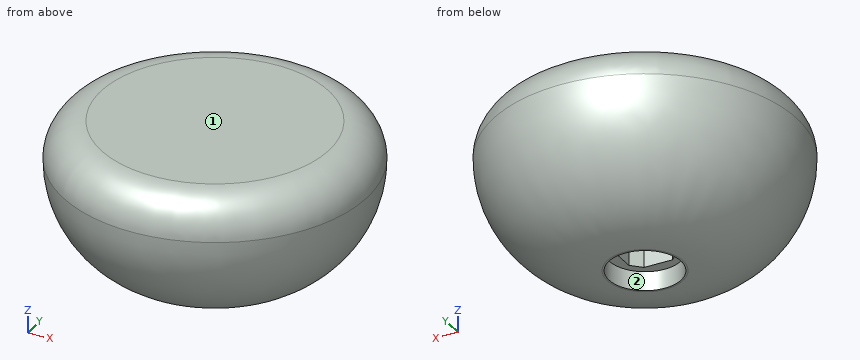
from build123d import *

# Parameters (mm, degrees)
EXTRUDE_3_OUTLINE_R   = 8
EXTRUDE_3_OUTLINE_R_2 = 1.904306864
EXTRUDE_3_OUTLINE_R_3 = 1.884306864
EXTRUDE_3_DEPTH       = 4
EXTRUDE_START         = -1
SKETCH_4_3_R          = 8
SKETCH_4_3_R_2        = 1.904306864
EXTRUDE_4_DEPTH       = 1
SKETCH_5_R            = 8
EXTRUDE_5_DEPTH       = 3
FILLET_3_R            = 2
FILLET_4_R            = 6


# Read off the part's stored shape, not the designer's step: 凸台-拉伸3
with BuildPart() as part:
    # 凸台-拉伸3 outline → 凸台-拉伸3 (new body)
    # profile 1 of 2: a face of its own
    with BuildSketch(Plane.XY.offset(15.156605354)):
        with Locations((62.088098202, 10.274465036)):
            Circle(EXTRUDE_3_OUTLINE_R)
        with Locations((62.088098202, 10.274465036)):
            Circle(EXTRUDE_3_OUTLINE_R_2, mode=Mode.SUBTRACT)
    # profile 2 of 2: a face of its own
    with BuildSketch(Plane.XY.offset(15.156605354)):
        with Locations((62.088098202, 10.274465036)):
            Circle(EXTRUDE_3_OUTLINE_R_3)
        Polygon((62.846382474, 11.544465036), (63.358098202, 11.032749307), (63.358098202, 9.516180765), (62.846382474, 9.004465036), (61.329813931, 9.004465036), (60.818098202, 9.516180765), (60.818098202, 11.032749307), (61.329813931, 11.544465036), align=None, mode=Mode.SUBTRACT)
    extrude(amount=EXTRUDE_3_DEPTH)

    # 草图4<3> → 凸台-拉伸4 (add)
    with BuildSketch(Plane.XY.offset(15.156605354).offset(EXTRUDE_START)):
        with Locations((62.088098202, 10.274465036)):
            Circle(SKETCH_4_3_R)
        with Locations((62.088098202, 10.274465036)):
            Circle(SKETCH_4_3_R_2, mode=Mode.SUBTRACT)
    extrude(amount=EXTRUDE_4_DEPTH)

    # 草图5 → 凸台-拉伸5 (add)
    with BuildSketch(Plane.XY.offset(19.156605354)):
        with Locations((62.088098202, 10.274465036)):
            Circle(SKETCH_5_R)
    extrude(amount=EXTRUDE_5_DEPTH)

    # 圆角3
    fillet_3_edges = [part.edges().sort_by_distance(p)[0] for p in [
        (54.088098202, 10.274465036, 22.156605354),
    ]]
    fillet(fillet_3_edges, radius=FILLET_3_R)

    # 圆角4
    fillet_4_edges = [part.edges().sort_by_distance(p)[0] for p in [
        (54.088098202, 10.274465036, 14.156605354),
    ]]
    fillet(fillet_4_edges, radius=FILLET_4_R - 0.0001)  # a hair under: the kernel refuses the full size


solid = part.part
Design review of the part built by this model. Coordinates are the model's own, in mm. Face numbers are marked on the shaded views. Give positions to 0.01 mm unless a question says otherwise; leave off trailing zeros. Loops run counter-clockwise (first coordinate to the right, second up) from the corner with the lowest first, then second, coordinate; pieces in that order, holes last. Notation, with made-up numbers: (-27, 82) - (17, 82) arc R25 ccw to (17, 97) - close; hole circle Ø8 at (32, 20.25). An arc over 180 degrees is marked (long way). Use CSV: the item, a comma, the result in double quotes. Start each with the question number.
1. Draft analysis for pull direction Y (two halves, no side actions). For the marked faces 1 and 2, state which applies: released by +Y, released by -Y, zero draft, split by the parting line, or undercut.
2. Add section A-A (z = 18.5). Count the separate pieces of the cut face and the enclosed holes in it, plus the area to 3 significant figures.
3. Wall thickness on L1, parallel to Z at x = 68, y = 9.75; L2, parallel to Z at x = 58.5, y = 10.25; L3, parallel to Y at x = 64.5, z = 21.75: over which ranges is each line inside the solid? List them lowest first.
4. Add section C-C (z = 21). State the section outline as (x, y) points.
5. Insertion check: P1, Ø1.7, axis at y = 10, z = 18, coming from the +X side; P2, Ø1.2, axis at y = 10, z = 17, coming from the -X side; P3, Ø0.5, axis at x = 62.5, z = 18, coming from the +Y side. Each pin has a flat end and moves straight along its axis. Give the tip position at first contact, or say it passes through.
Results found:
1,face 1,"zero draft"
1,face 2,"undercut"
2,separate pieces,"2"
2,enclosed holes,"2"
2,area,"183 mm²"
3,L1,"z = 15.63 to 22.16"
3,L2,"z = 14.37 to 22.16"
3,L3,"y = 3.48 to 17.07"
4,outline,"circle Ø15.63 at (62.09, 10.27)"
5,P1,"stops at x = 69.94"
5,P2,"stops at x = 54.66"
5,P3,"stops at y = 17.95"
